from build123d import *

# Parameters (mm, degrees)
SKETCH2_W           = 55
SKETCH2_H           = 6
BOSS_EXTRUDE8_DEPTH = 5
SKETCH4_R           = 0.3
CUT_EXTRUDE3_DEPTH  = 2
SKETCH5_R           = 0.3
CUT_EXTRUDE4_DEPTH  = 2
SKETCH6_R           = 1.5
CUT_EXTRUDE5_DEPTH  = 10


with BuildPart() as part:
    # Sketch2 → Boss-Extrude8 (new body)
    with BuildSketch(Plane.XY):
        with Locations((0, -3)):
            Rectangle(SKETCH2_W, SKETCH2_H)
        with BuildLine():
            ThreePointArc((-27.5, -6), (-30.328427125, -7.171572875), (-31.5, -10))
            Line((-31.5, -10), (-31.5, -12))
            Line((-31.5, -12), (-33.5, -12))
            Line((-33.5, -12), (-33.5, -6))
            ThreePointArc((-33.5, -6), (-31.742640687, -1.757359313), (-27.5, 0))
            Line((-27.5, 0), (-27.5, -6))
        make_face()
        with BuildLine():
            Line((27.5, -6), (27.5, 0))
            ThreePointArc((27.5, 0), (31.742640687, -1.757359313), (33.5, -6))
            Line((33.5, -6), (33.5, -12))
            Line((33.5, -12), (31.5, -12))
            Line((31.5, -12), (31.5, -10))
            ThreePointArc((31.5, -10), (30.328427125, -7.171572875), (27.5, -6))
        make_face()
    extrude(amount=BOSS_EXTRUDE8_DEPTH)

    # Sketch4 → Cut-Extrude3 (cut)
    with BuildSketch(Plane(origin=(33.5, 0, 0), x_dir=(0, 0, -1), z_dir=(1, 0, 0))):
        with Locations((-4, -11)):
            Circle(SKETCH4_R)
    extrude(amount=-CUT_EXTRUDE3_DEPTH, mode=Mode.SUBTRACT)

    # Sketch5 → Cut-Extrude4 (cut)
    with BuildSketch(Plane.ZY.offset(33.5)):
        with Locations((1, -11)):
            Circle(SKETCH5_R)
    extrude(amount=-CUT_EXTRUDE4_DEPTH, mode=Mode.SUBTRACT)

    # Sketch6 → Cut-Extrude5 (cut)
    with BuildSketch(Plane(origin=(0, 0, 0), x_dir=(1, 0, 0), z_dir=(0, 1, 0))):
        with Locations(Location((-20, -2.45, 0), (0, 0, 270))):
            Circle(SKETCH6_R)
        with Locations(Location((20, -2.45, 0), (0, 0, 270))):
            Circle(SKETCH6_R)
    extrude(amount=-CUT_EXTRUDE5_DEPTH, mode=Mode.SUBTRACT)


solid = part.part
Could you check a few things on this model? Use its own coordinates, in mm. A direction names the side the tool comes from. Give positions to 0.01 mm unless a question says otherwise; leave off trailing zeros. Order: outer loops, then holes, each group sorted by start corner. A loop starts at its lowest first (then second) coordinate and runs counter-clockwise, first axis right, second up. Notation, with made-up numbers: (-8, -3) - (13, -3) arc R16 cw to (13, 6) - close; hole circle Ø11 at (64, 19). An arc over 180 degrees is marked (long way). Return JSON: item names as keys, results as strings. Group by question number.
Q1. Suppose I cut it at D-D, the plane x = 12. Please give me the cut outline in (y, z).
Q2. Suppose I cut it at A-A, the plane z = 2.45. Please give me the cut outline in (x, y), and give its area (3 significant figures).
Q3. Will these pins go through, and if not, where does the flat tip stop? pin 1 Ø1 at (y, z) = (-3.5, 3) entering from -X; pin 2 Ø1.5 at (x, z) = (-9.5, 1.5) entering from -Y.
Q4. Suppose I cut it at C-C, the plane y = -0.75. Please give me the cut outline in (x, z).
Q5. Suppose I cut it at B-B, the plane x = -20. Please give me the cut outline in (y, z).
Q6. Thinking about a two-plate mould opening in Z: for faces 1 (the face through (30.359, -7.203, 2.465)), 2 (the face through (21.265, -2.958, 3.256)), 3 (the face through (0, -3, 0)), which applies, pulls with the +Z half, pulls with the -Z half, needs draft (parallel to the pull), parting line crosses it, or undercut?
Q7. Which directions (+Z, -Z, +X, -X, +Y, -Y) give clear straight access to the entire face, cutting with the end or side of a thin tool? Please do faces 4 (the face through (-30.297, -7.141, 2.465)), 5 (the face through (-18.735, -2.958, 3.256)).
Q8. Please list where these lines run through material, in increasing order: line 1 along X through (y, z) = (-4.75, 3.65); line 2 along Y through (x, z) = (-21, 1.05); line 3 along X through (y, z) = (-10.25, 1.65). Write a range as [from, to].
Resolved:
{
 "1": {"outline": "(-6, 0) - (0, 0) - (0, 5) - (-6, 5) - close"},
 "2": {"outline": "(-33.5, -12) - (-31.5, -12) - (-31.5, -10) arc R4 cw to (-27.5, -6) - (-21.5, -6) - (-21.5, 0) - (-27.5, 0) arc R6 ccw to (-33.5, -6) - close; (-18.5, -6) - (18.5, -6) - (18.5, 0) - (-18.5, 0) - close; (21.5, -6) - (27.5, -6) arc R4 cw to (31.5, -10) - (31.5, -12) - (33.5, -12) - (33.5, -6) arc R6 ccw to (27.5, 0) - (21.5, 0) - close", "area": "381 mm2"},
 "3": {"pin 1": "stops at x = -33.16", "pin 2": "stops at y = -6"},
 "4": {"outline": "(-30.4, 0) - (30.4, 0) - (30.4, 5) - (-30.4, 5) - close; hole circle Ø3 at (-20, 2.45); hole circle Ø3 at (20, 2.45)"},
 "5": {"outline": "(-6, 0) - (0, 0) - (0, 0.95) - (-6, 0.95) - close; (-6, 3.95) - (0, 3.95) - (0, 5) - (-6, 5) - close"},
 "6": {"face 1": "needs draft", "face 2": "undercut", "face 3": "pulls with the -Z half"},
 "7": {"face 4": "+Z, -Z, -Y", "face 5": "+Y, -Y"},
 "8": {"line 1": "x = [-33.37, -20.9], [-19.1, 19.1], [20.9, 33.37]", "line 2": "y = [-6, 0]", "line 3": "x = [-33.5, -31.5], [31.5, 33.5]"}
}
